Verification items for the finished model (mm, model axes). Face numbers are marked on the shaded views. A direction names the side the tool comes from. Coordinates: 2 decimals unless noted, no trailing zeros. Write each loop counter-clockwise with the first axis right and the second up, starting at its lowest first coordinate (ties: lowest second). Pieces come first, ordered by that corner, then holes.
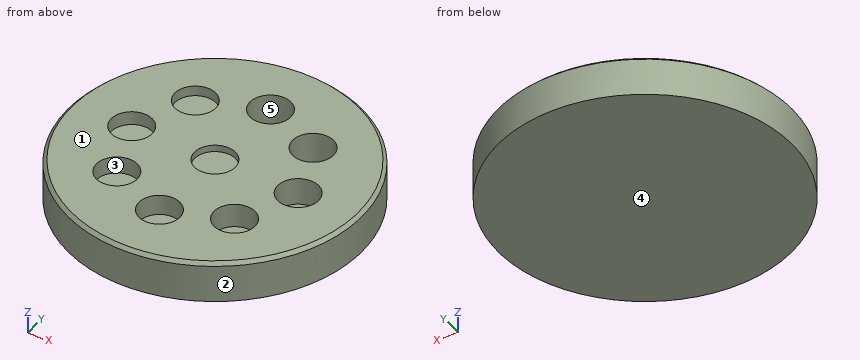
Autodesk Inventor part; units mm, degrees
ref_plane "YZ Plane" through (0, 0, 0) normal (1, 0, 0) x (0, 1, 0)
ref_plane "XZ Plane" through (0, 0, 0) normal (0, 1, 0) x (-1, 0, 0)
ref_plane "XY Plane" through (0, 0, 0) normal (0, 0, 1) x (1, 0, 0)
sketch "Sketch1" plane through (0, 0, 0) normal (0, 0, 1) x (1, 0, 0)
  circle A0 centre (0, 0) radius 43
  circle A1 centre (0, 0) radius 6
  circle A2 centre (0, 25) radius 6
  circle A3 centre (-17.6777, 17.6777) radius 6
  circle A4 centre (-25, 0) radius 6
  circle A5 centre (-17.6777, -17.6777) radius 6
  circle A6 centre (0, -25) radius 6
  circle A7 centre (17.6777, -17.6777) radius 6
  circle A8 centre (25, 0) radius 6
  circle A9 centre (17.6777, 17.6777) radius 6
  dimension "diameter" = 12
  dimension "d2" = 12
  dimension "d5" = 360
  dimension "d7" = 25
  dimension "d28" = 86
extrude "Extrusion1" add sketch "Sketch1" along normal blind 12
extrude "Extrusion2" add sketch "Sketch1" along normal blind 2 contours A2
extrude "Extrusion3" add sketch "Sketch1" along normal blind 3 contours A9
extrude "Extrusion4" add sketch "Sketch1" along normal blind 4 contours A8
extrude "Extrusion5" add sketch "Sketch1" along normal blind 5 contours A7
extrude "Extrusion6" add sketch "Sketch1" along normal blind 6 contours A6
extrude "Extrusion7" add sketch "Sketch1" along normal blind 7 contours A5
extrude "Extrusion8" add sketch "Sketch1" along normal blind 8 contours A4
extrude "Extrusion9" add sketch "Sketch1" along normal blind 9 contours A3
extrude "Extrusion10" add sketch "Sketch1" along normal blind 10 contours A1
sketch "Sketch2" plane through (0, 0, 12) normal (0, 0, 1) x (1, 0, 0)
  line L0 (-5.8774, 39.105) -> (5.7366, 39.105) construction
  line L1 (5.7366, 39.105) -> (5.7366, 35.936) construction
  line L2 (5.7366, 35.936) -> (-5.8774, 35.936) construction
  line L3 (-5.8774, 35.936) -> (-5.8774, 39.105) construction
  point P0 (0, 0)
emboss "Emboss1" [suppressed]
chamfer "Chamfer1" distance 1 angle 45 1 edges at (-43, 0, 12)
equation "\"d2\" = diameter"
properties part number "Diameter_12mm"
1. Tool access check on the marked faces 4 and 5. Record the directions out of +Z, -Z, +X, -X, +Y, -Y that give a thin tool (end or side, any length) a straight path to the whole face; none if there is none.
2. Gauge pin test, flat ends, axial feed: P1, Ø3.5, axis at x = 18, y = -15, coming from the +Z side; P2, Ø6, axis at x = -15.5, y = -16.5, coming from the +Z side; P3, Ø3.5, axis at x = 16, y = 20.5, coming from the +Z side. Record the tip position at first contact, or that the pin passes through.
3. Material ranges on L1, parallel to Y at x = 0, z = 4.25; L2, parallel to Y at x = 15, z = 11; L3, parallel to X at y = 25.5, z = 3.25, recorded low to high.
4. Sectioned sample at A-A, the plane x = 0. Record the boundary of the cut face in (y, z).
5. Draft check along Y on the marked faces 1, 2 and 3. Enter one of: pulls with the +Y half, pulls with the -Y half, needs draft (parallel to the pull), parting line crosses it, or undercut.
6. Sectioned sample at B-B, the plane y = 0. Record the boundary of the cut face in (x, z), and give its area (3 significant figures).
Outcome:
1. face 4: -Z, +X, -X, +Y, -Y
1. face 5: +Z
2. P1: stops at z = 5
2. P2: stops at z = 7
2. P3: stops at z = 3
3. L1: y = -43 to 19, 31 to 43
3. L2: y = -40.3 to -23.05, -12.31 to 12.31, 23.05 to 40.3
3. L3: x = -34.62 to -5.98, 5.98 to 34.62
4. outline: (-43, 0) - (43, 0) - (43, 11) - (42, 12) - (31, 12) - (31, 2) - (19, 2) - (19, 12) - (6, 12) - (6, 10) - (-6, 10) - (-6, 12) - (-19, 12) - (-19, 6) - (-31, 6) - (-31, 12) - (-42, 12) - (-43, 11) - close
5. face 1: needs draft
5. face 2: parting line crosses it
5. face 3: undercut
6. outline: (-43, 0) - (43, 0) - (43, 11) - (42, 12) - (31, 12) - (31, 4) - (19, 4) - (19, 12) - (6, 12) - (6, 10) - (-6, 10) - (-6, 12) - (-19, 12) - (-19, 8) - (-31, 8) - (-31, 12) - (-42, 12) - (-43, 11) - close
6. area: 863 mm2
